Can you work these out from the drawing? Everything is in mm from the part's minimum corner. Give positions to 0.01 mm unless a question says otherwise; leave off trailing zeros. Write each loop counter-clockwise with the first axis right and the second up, starting at its lowest first coordinate (ties: lowest second). Pieces come first, ordered by that corner, then holes. Notation, with made-up numbers: (71, -14) -> (97, -14) arc R33 ccw to (97, 20) -> close; hole circle Ø6 at (31.25, -18). An arc over 180 degrees is marked (long way). Return JSON: item names as keys, results as strings.
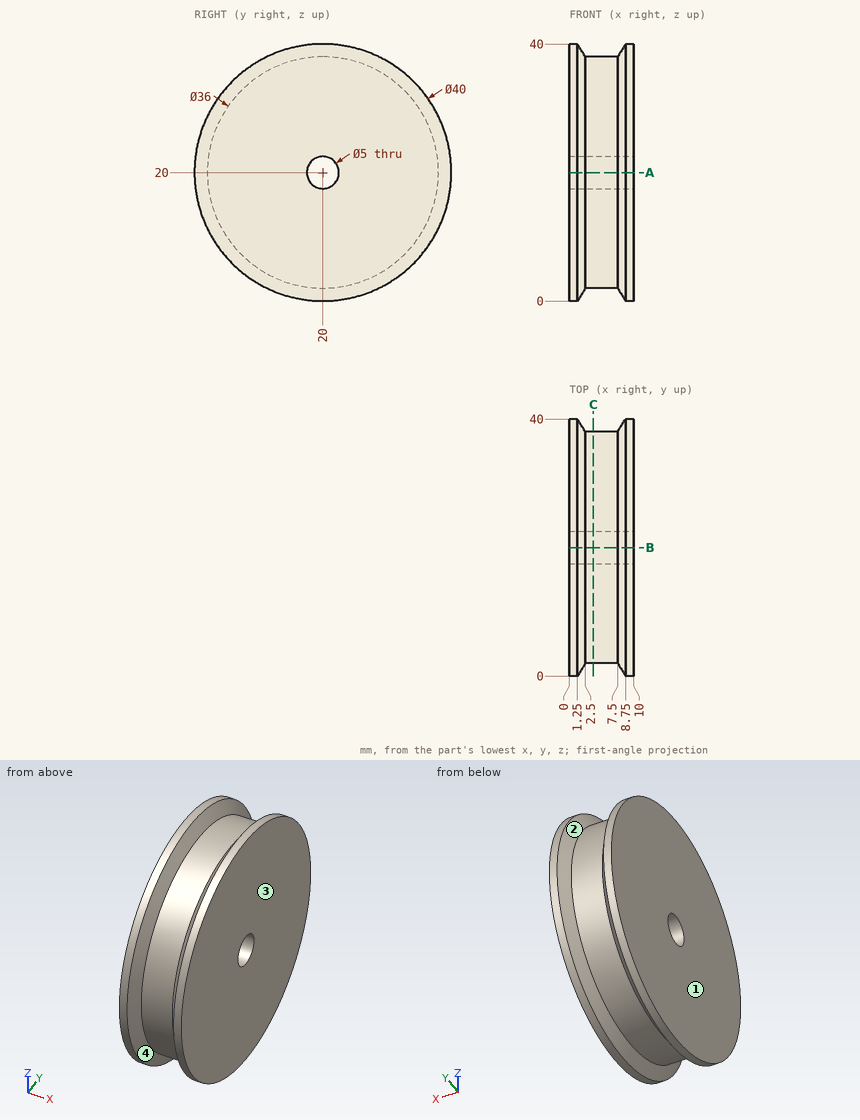
1. If I drill on line 1 (Y direction, x = 5, z = 20); line 2 (Z direction, x = 8.5, y = 20), over which ranges is the centre line in solid material (lowest first)? Write a range as [from, to].
Taken from the geometry:
{"line 1": "y = [2, 17.5], [22.5, 38]", "line 2": "z = [0.4, 17.5], [22.5, 39.6]"}
2. Suppose I cut it at A-A, the plane z = 20. List the corners of the cut face in (x, y) for me, and give its area (3 significant figures).
Taken from the geometry:
{"outline": "(0, 0) -> (1.25, 0) -> (2.5, 2) -> (7.5, 2) -> (8.75, 0) -> (10, 0) -> (10, 17.5) -> (0, 17.5) -> close; (0, 22.5) -> (10, 22.5) -> (10, 40) -> (8.75, 40) -> (7.5, 38) -> (2.5, 38) -> (1.25, 40) -> (0, 40) -> close", "area": "325 mm²"}
3. For pin 1 Ø6 at (x, y) = (1.5, 9.5) entering from +Z; pin 2 Ø5 at (x, z) = (8.5, 25.5) entering from -Y; pin 3 Ø3 at (x, y) = (7.5, 10) entering from +Z, each with a flat end and sliding along its axis, tell me the tip position at first contact or that it passes through.
Taken from the geometry:
{"pin 1": "stops at z = 38.54", "pin 2": "stops at y = 0.23", "pin 3": "stops at z = 37.77"}
4. If we mould it in two halves opening along X, with no side actions, what happens to the marked faces 1, 2, 3 and 4? For each: released by +X, released by -X, zero draft, split by the parting line, or undercut.
Taken from the geometry:
{"face 1": "released by -X", "face 2": "undercut", "face 3": "released by +X", "face 4": "undercut"}
5. Suppose I cut it at C-C, the plane x = 3.75. List the corners of the cut face in (y, z) for me, and give its area (3 significant figures).
Taken from the geometry:
{"outline": "circle Ø36 at (20, 20); hole circle Ø5 at (20, 20)", "area": "998 mm²"}
